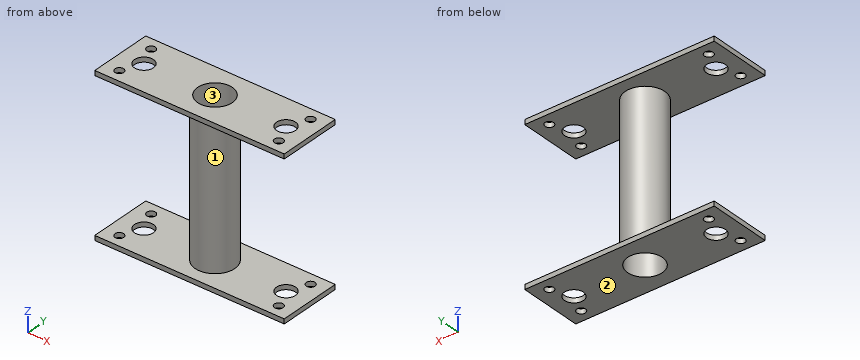
from build123d import *

# Parameters (mm, degrees)
SKETCH_1_W               = 120
SKETCH_1_H               = 40
EXTRUDE_1_DEPTH          = 3
SKETCH_2_R               = 12.5
EXTRUDE_2_DEPTH          = 94
SKETCH_3_W               = 120
SKETCH_3_H               = 40
EXTRUDE_3_DEPTH          = 3
CUT_EXTRUDE_1_DEPTH      = 119.321595662
CUT_EXTRUDE_1_DEPTH_BACK = 119.321595662
SKETCH_4_R               = 11
SKETCH_5_R               = 2.75
CUT_EXTRUDE_2_DEPTH      = 119.321595662
SKETCH_6_R               = 6
CUT_EXTRUDE_3_DEPTH      = 119.321595662


with BuildPart() as part:
    # 草图1 → 凸台-拉伸1 (new body)
    with BuildSketch(Plane.XY):
        Rectangle(SKETCH_1_W, SKETCH_1_H)
    extrude(amount=EXTRUDE_1_DEPTH)

    # 草图2 → 凸台-拉伸2 (add)
    with BuildSketch(Plane.XY.offset(3)):
        Circle(SKETCH_2_R)
    extrude(amount=EXTRUDE_2_DEPTH)

    # 草图3 → 凸台-拉伸3 (add)
    with BuildSketch(Plane.XY.offset(97)):
        Rectangle(SKETCH_3_W, SKETCH_3_H)
    extrude(amount=EXTRUDE_3_DEPTH)

    # 草图4 → 切除-拉伸1 (cut, two sides: drawn at the far end of the back side and taken through both)
    with BuildSketch(Plane.XY.offset(100).offset(-CUT_EXTRUDE_1_DEPTH_BACK)):
        Circle(SKETCH_4_R)
    extrude(amount=CUT_EXTRUDE_1_DEPTH + CUT_EXTRUDE_1_DEPTH_BACK, mode=Mode.SUBTRACT)

    # 草图5 → 切除-拉伸2 (cut, through all)
    with BuildSketch(Plane.XY.offset(100)):
        with Locations((-50.5, 12.5)):
            Circle(SKETCH_5_R)
        with Locations((-50.5, -12.5)):
            Circle(SKETCH_5_R)
        with Locations((50.5, 12.5)):
            Circle(SKETCH_5_R)
        with Locations((50.5, -12.5)):
            Circle(SKETCH_5_R)
    extrude(amount=-CUT_EXTRUDE_2_DEPTH, mode=Mode.SUBTRACT)

    # 草图6 → 切除-拉伸3 (cut, through all)
    with BuildSketch(Plane.XY.offset(100)):
        with Locations((45, 0)):
            Circle(SKETCH_6_R)
        with Locations((-45, 0)):
            Circle(SKETCH_6_R)
    extrude(amount=-CUT_EXTRUDE_3_DEPTH, mode=Mode.SUBTRACT)


solid = part.part
Input: part model. Units: mm. Frame: model coordinates. Face numbers are marked on the shaded views. Give positions to 0.01 mm unless a question says otherwise; leave off trailing zeros. Write each loop counter-clockwise with the first axis right and the second up, starting at its lowest first coordinate (ties: lowest second). Pieces come first, ordered by that corner, then holes. Notation, with made-up numbers: (74, 45.5) -> (93, 45.5) arc R3 ccw to (93, 50.5) -> close; hole circle Ø8 at (27, 43). An arc over 180 degrees is marked (long way). Use one line per item in the form item = value. Start each with the question number.
1) Section query B-B on y = 0. Count the separate pieces of the cut face and the enclosed holes in it, then the cut area to 3 significant figures.
2) Draft query along X for the marked faces 1, 2 and 3. Return one class per face: pulls with the +X half, pulls with the -X half, needs draft (parallel to the pull), parting line crosses it, or undercut.
3) Pin query (flat end, axial travel): pin 1 (6 mm diameter, centred on x = -5, z = 25.5, fed in from +Y); pin 2 (6 mm diameter, centred on y = 3.5, z = 48, fed in from -X); pin 3 (1.5 mm diameter, centred on y = -10, z = 44.5, fed in from -X). Return the tip coordinate at first contact, or that it passes through.
4) Section query A-A on x = 0. Return the cut outline in (y, z).
5) Section query D-D on x = 25. Return the cut outline in (y, z), then the cut area to 3 significant figures.
6) Section query C-C on x = -45. Return the cut outline in (y, z), then the cut area to 3 significant figures.
7) Ray query, probe 1 along Z at (x, y) = (16.5, -0.5); probe 2 along Y at (x, z) = (-45, 1.7); probe 3 along Y at (x, z) = (-50.5, 98.15). Return the intervals inside material, ascending. Write a range as from..to.
Outcome:
q1.separate_pieces = 6
q1.enclosed_holes = 0
q1.area = 726 mm^2
q2.face_1 = parting line crosses it
q2.face_2 = needs draft
q2.face_3 = undercut
q3.pin_1 = 12.34
q3.pin_2 = -12.49
q3.pin_3 = -8.41
q4.outline = (-20, 0) -> (-11, 0) -> (-11, 100) -> (-20, 100) -> (-20, 97) -> (-12.5, 97) -> (-12.5, 3) -> (-20, 3) -> close; (11, 0) -> (20, 0) -> (20, 3) -> (12.5, 3) -> (12.5, 97) -> (20, 97) -> (20, 100) -> (11, 100) -> close
q5.outline = (-20, 0) -> (20, 0) -> (20, 3) -> (-20, 3) -> close; (-20, 97) -> (20, 97) -> (20, 100) -> (-20, 100) -> close
q5.area = 240 mm^2
q6.outline = (-20, 0) -> (-6, 0) -> (-6, 3) -> (-20, 3) -> close; (-20, 97) -> (-6, 97) -> (-6, 100) -> (-20, 100) -> close; (6, 0) -> (20, 0) -> (20, 3) -> (6, 3) -> close; (6, 97) -> (20, 97) -> (20, 100) -> (6, 100) -> close
q6.area = 168 mm^2
q7.probe_1 = 0..3, 97..100
q7.probe_2 = -20..-6, 6..20
q7.probe_3 = -20..-15.25, -9.75..-2.4, 2.4..9.75, 15.25..20
